Read the model definition and answer for the solid it produces. Units are mm, in the model's axes. Face numbers are marked on the shaded views. A direction names the side the tool comes from. Coordinates: 2 decimals unless noted, no trailing zeros. Loops run counter-clockwise (first coordinate to the right, second up) from the corner with the lowest first, then second, coordinate; pieces in that order, holes last. Notation, with made-up numbers: (62, 23.5) -> (102, 23.5) arc R16 cw to (102, 32.5) -> close; hole circle Ø9 at (-8, 40.25). An arc over 180 degrees is marked (long way). Answer as a JSON object with one key per item and string values. Group by question number.
Q1. The part is cut by section A-A on x = -19.5. Write down the section's boundary in (y, z).
Q2. Straight lines are drawn through the part: line 1 along Z through (x, y) = (-11.5, 35); line 2 along Z through (x, y) = (-52, 5). For each, find the intervals that lie inside material, in ascending order. Write a range as [from, to].
Q3. For the marked faces 4, 5 and 6, determine the directions among +Z, -Z, +X, -X, +Y, -Y from which every point of the face is accessible in a straight line to the end or side of a thin tool.
Q4. The part is cut by section C-C on z = -84. Write down the section's boundary in (x, y), and give its area (3 significant figures).
Q5. Determine the mould class of the marked faces 1, 2 and 3 for opening direction Z: released by +Z, released by -Z, zero draft, split by the parting line, or undercut.
Q6. The part is cut by section B-B on y = 75.5. Write down the section's boundary in (x, z), and give its area (4 significant figures).
Q7. Each of these flat-tipped pins is pushed along its axis until it touches: P1, Ø5.5, axis at y = 44, z = -216.5, coming from the -X side; P2, Ø20, axis at y = 63.5, z = -21, coming from the +X side; P3, Ø4, axis at y = 87.5, z = -146, coming from the -X side; P4, Ø2.5, axis at x = -97.5, y = 56.5, coming from the -Z side. Where does it stop, or does it pass through?
Q8. The part is cut by section D-D on x = -73.5. Write down the section's boundary in (y, z), and give its area (3 significant figures).
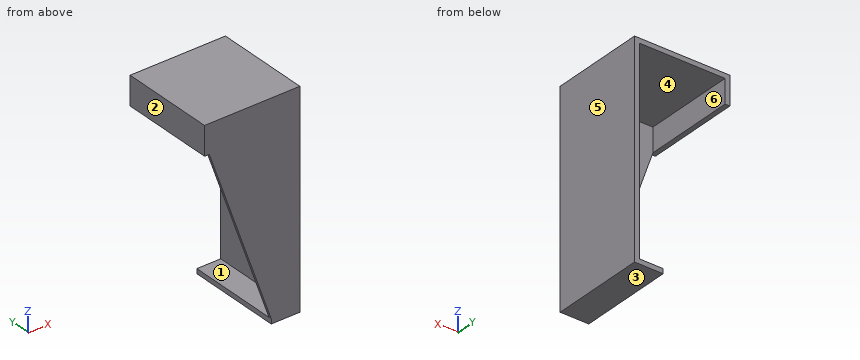
from build123d import *

# Parameters (mm, degrees)
ESTRUSIONE_ESTRUSIONE1_DEPTH = 100
ESTRUSIONE_ESTRUSIONE2_DEPTH = 3


with BuildPart() as part:
    # Schizzo1 → Estrusione-Estrusione1 (new body)
    with BuildSketch(Plane(origin=(0, 0, 0), x_dir=(1, 0, 0), z_dir=(0, 1, 0))):
        Polygon((-100, 0), (0, 0), (0, 220), (-30, 220), (-30, 215), (-5, 215), (-5, 5), (-95, 5), (-95, 30), (-100, 30), align=None)
    extrude(amount=ESTRUSIONE_ESTRUSIONE1_DEPTH)

    # Schizzo2 → Estrusione-Estrusione2 (add)
    with BuildSketch(Plane.XZ):
        Polygon((-30, -215), (-5, -215), (-5, -5), (-95, -5), (-95, -30), align=None)
    extrude(amount=-ESTRUSIONE_ESTRUSIONE2_DEPTH)


solid = part.part
Final values:
{
 "1": {"outline": "(0, -220) -> (100, -220) -> (100, -215) -> (3, -215) -> (3, -5) -> (100, -5) -> (100, 0) -> (0, 0) -> close"},
 "2": {"line 1": "z = [-220, -215], [-5, 0]", "line 2": "z = [-5, 0]"},
 "3": {"face 4": "+Y", "face 5": "+Z, -Z, +X, +Y, -Y", "face 6": "-Z, +Y"},
 "4": {"outline": "(-76.03, 0) -> (0, 0) -> (0, 100) -> (-5, 100) -> (-5, 3) -> (-76.03, 3) -> close", "area": "713 mm2"},
 "5": {"face 1": "undercut", "face 2": "zero draft", "face 3": "released by -Z"},
 "6": {"outline": "(-100, -30) -> (-95, -30) -> (-95, -5) -> (-5, -5) -> (-5, -215) -> (-30, -215) -> (-30, -220) -> (0, -220) -> (0, 0) -> (-100, 0) -> close", "area": "1,825 mm2"},
 "7": {"P1": "stops at x = -30", "P2": "stops at x = 0", "P3": "stops at x = -5", "P4": "stops at z = -30"},
 "8": {"outline": "(0, -91.19) -> (3, -91.19) -> (3, -5) -> (100, -5) -> (100, 0) -> (0, 0) -> close", "area": "759 mm2"}
}
